Verification items for the finished model (mm, model axes). Face numbers are marked on the shaded views. A direction names the side the tool comes from. Coordinates: 2 decimals unless noted, no trailing zeros. Order: outer loops, then holes, each group sorted by start corner. A loop starts at its lowest first (then second) coordinate and runs counter-clockwise, first axis right, second up. Notation, with made-up numbers: M 20.25,56.5 L 75.25,56.5 A8 cw 75.25,70.5 Z; hole C 4.25,6.25 d11. An arc over 180 degrees is marked long. Return JSON: item names as keys, results as strings.
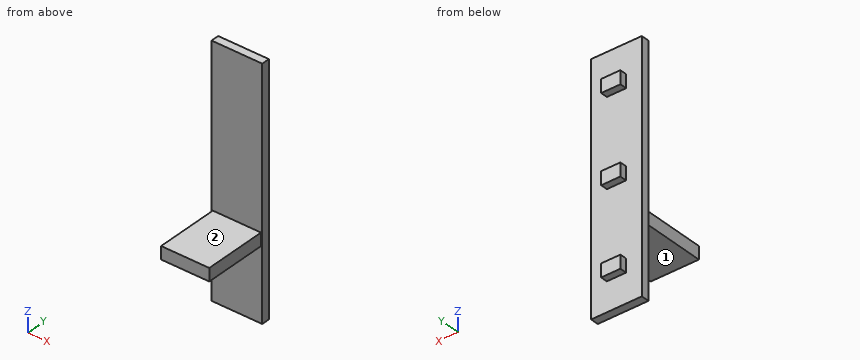
Autodesk Inventor part; units mm, degrees
ref_plane "YZ Plane" through (0, 0, 0) normal (1, 0, 0) x (0, 1, 0)
ref_plane "XZ Plane" through (0, 0, 0) normal (0, 1, 0) x (-1, 0, 0)
ref_plane "XY Plane" through (0, 0, 0) normal (0, 0, 1) x (1, 0, 0)
sketch "Sketch2" plane through (0, 0, 0) normal (0, 1, 0) x (-1, 0, 0)
  line L0 (10, 0) -> (0, 0)
  line L1 (0, 0) -> (0, -48)
  line L2 (0, -48) -> (10, -48)
  line L3 (10, -48) -> (10, 0)
  line L4 (6.9, -8.3) -> (3.1, -8.3)
  line L5 (3.1, -8.3) -> (3.1, -5.7)
  line L6 (3.1, -5.7) -> (6.9, -5.7)
  line L7 (6.9, -5.7) -> (6.9, -8.3)
  line L8 (6.9, -39.7) -> (3.1, -39.7)
  line L9 (3.1, -39.7) -> (3.1, -42.3)
  line L10 (3.1, -42.3) -> (6.9, -42.3)
  line L11 (6.9, -42.3) -> (6.9, -39.7)
  line L12 (3.1, -22.7) -> (6.9, -22.7)
  line L13 (3.1, -25.3) -> (3.1, -22.7)
  line L14 (6.9, -25.3) -> (3.1, -25.3)
  line L15 (6.9, -22.7) -> (6.9, -25.3)
  line L16 (23.6892, -32.5) -> (-2.3247, -32.5) construction
  line L17 (5, -54.7987) -> (5, -48.1542) construction
  line L18 (5, 9.3713) -> (5, -46.1174) construction
  line L19 (11.7769, -7) -> (1.25, -7) construction
  line L20 (11.7769, -24) -> (1.25, -24) construction
  line L21 (11.7769, -41) -> (1.25, -41) construction
  line L22 (9.75, -31.25) -> (0.25, -31.25)
  line L23 (0.25, -33.75) -> (9.75, -33.75)
  line L24 (9.75, -31.25) -> (9.75, -33.75)
  line L25 (0.25, -31.25) -> (0.25, -33.75)
  dimension "d0" = 10
  dimension "d1" = 48
  dimension "d13" = 3.8
  dimension "d14" = 2.6
  dimension "d40" = 5
  dimension "d49" = 15.5
  dimension "d50" = 7
  dimension "d51" = 24
  dimension "d52" = 41
  dimension "d53" = 2.5
  dimension "d54" = 9.5
extrude "Extrusion1" add sketch "Sketch2" along normal blind 1.6 contours L3 L2 L1 L0 | L4 L5 L6 L7 | L11 L10 L9 L8 | L12 L15 L14 L13 | L24 L23 L25 L22
extrude "Extrusion4" add sketch "Sketch2" along normal blind 2.98 contours L4 L5 L6 L7 | L11 L10 L9 L8 | L12 L15 L14 L13
sketch "Sketch3" plane through (0, 2.98, 0) normal (0, 1, 0) x (1, 0, 0)
  line L0 (-3.1, 25.3) -> (-6.9, 25.3) construction
  line L1 (-6.9, 22.7) -> (-3.1, 22.7) construction
  point P0 (0, 0)
  point P1 (-5.1459, 24.0493)
extrude "Extrusion5" add sketch "Sketch2" against normal blind 12.5 contours L24 L23 L25 L22
properties part number "Sensor_Board_dummy"
Q1. Tool access check on the marked faces 1 and 2. Record the directions out of +Z, -Z, +X, -X, +Y, -Y that give a thin tool (end or side, any length) a straight path to the whole face; none if there is none.
Values:
{"face 1": "-Z, +X, -X, -Y", "face 2": "+Z, +X, -X, -Y"}
Q2. Cross-section at B-B, the plane x = -6. Record the boundary of the cut face in (y, z).
Values:
{"outline": "M -12.5,-33.75 L 0,-33.75 L 0,-48 L 1.6,-48 L 1.6,-42.3 L 2.98,-42.3 L 2.98,-39.7 L 1.6,-39.7 L 1.6,-25.3 L 2.98,-25.3 L 2.98,-22.7 L 1.6,-22.7 L 1.6,-8.3 L 2.98,-8.3 L 2.98,-5.7 L 1.6,-5.7 L 1.6,0 L 0,0 L 0,-31.25 L -12.5,-31.25 Z"}
Q3. Go/stop test with flat-tipped pins: pin 1 (0.7 mm diameter, centred on y = 2, z = -6.5, fed in from +X); pin 2 (4 mm diameter, centred on x = -1, y = -7, fed in from -Z); pin 3 (0.7 mm diameter, centred on x = -4.5, y = 2, fed in from -Z); pin 4 (1.5 mm diameter, centred on y = -1, z = -13, fed in from +X). Record where each tip stops, or that it passes through.
Values:
{"pin 1": "x = -3.1", "pin 2": "z = -33.75", "pin 3": "z = -42.3", "pin 4": "through"}
Q4. Cross-section at D-D, the plane z = -38. Record the boundary of the cut face in (x, y).
Values:
{"outline": "M -10,0 L 0,0 L 0,1.6 L -10,1.6 Z"}
Q5. Cross-section at C-C, the plane x = -2. Record the boundary of the cut face in (y, z).
Values:
{"outline": "M -12.5,-33.75 L 0,-33.75 L 0,-48 L 1.6,-48 L 1.6,0 L 0,0 L 0,-31.25 L -12.5,-31.25 Z"}
Q6. Cross-section at A-A, the plane y = 2.25. Record the boundary of the cut face in (x, z), and give its area (3 significant figures).
Values:
{"outline": "M -6.9,-42.3 L -3.1,-42.3 L -3.1,-39.7 L -6.9,-39.7 Z; M -6.9,-25.3 L -3.1,-25.3 L -3.1,-22.7 L -6.9,-22.7 Z; M -6.9,-8.3 L -3.1,-8.3 L -3.1,-5.7 L -6.9,-5.7 Z", "area": "29.6 mm^2"}
Q7. Material ranges on line 1 along Z through (x, y) = (-4.75, 2); line 2 along Y through (x, z) = (-2.75, -26); line 3 along Z through (x, y) = (-8, -9.5), recorded low to high.
Values:
{"line 1": "-42.3 to -39.7, -25.3 to -22.7, -8.3 to -5.7", "line 2": "0 to 1.6", "line 3": "-33.75 to -31.25"}
